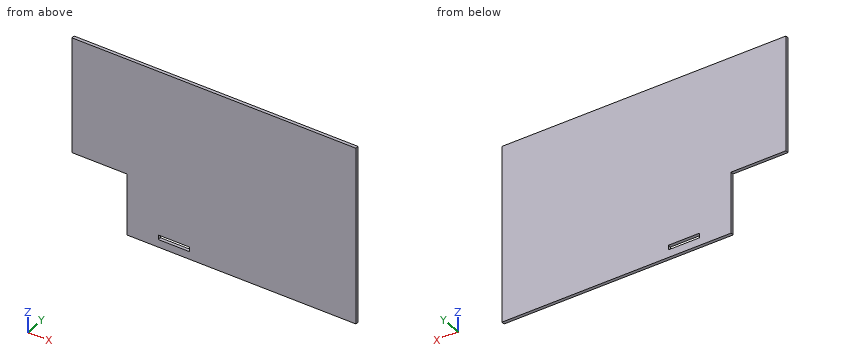
```python
from build123d import *

# Parameters (mm, degrees)
SKETCH1_W           = 25.4
SKETCH1_H           = 3.81
BOSS_EXTRUDE1_DEPTH = 2.54


with BuildPart() as part:
    # Sketch1 → Boss-Extrude1 (new body)
    with BuildSketch(Plane(origin=(0, 0, 0), x_dir=(1, 0, 0), z_dir=(0, 1, 0))):
        Polygon((0, -50.8), (44.45, -50.8), (44.45, 0), (229.87, 0), (229.87, -146.4056), (0, -146.4056), align=None)
        with Locations((82.55, -8.255)):
            Rectangle(SKETCH1_W, SKETCH1_H, mode=Mode.SUBTRACT)
    extrude(amount=BOSS_EXTRUDE1_DEPTH)


solid = part.part
```
Here's how the part is built. I have some questions about the finished solid (model axes, mm). Round coordinates to 2 decimals unless told otherwise and drop trailing zeros. Loops run counter-clockwise (first coordinate to the right, second up) from the corner with the lowest first, then second, coordinate; pieces in that order, holes last.
1. Suppose I cut it at C-C, the plane z = 32.5. Please give me the cut outline in (x, y).
Answers:
outline: (44.45, 0) - (229.87, 0) - (229.87, 2.54) - (44.45, 2.54) - close
2. Suppose I cut it at B-B, the plane x = 89. Please give me the cut outline in (y, z), and give its area (3 significant figures).
Answers:
outline: (0, 0) - (2.54, 0) - (2.54, 6.35) - (0, 6.35) - close; (0, 10.16) - (2.54, 10.16) - (2.54, 146.41) - (0, 146.41) - close
area: 362 mm2
3. Will these pins go through, and if not, where does the flat tip stop? pin 1 (0.8 mm diameter, centred on x = 81, y = 1.5, fed in from -Z); pin 2 (0.8 mm diameter, centred on x = 22.5, y = 2, fed in from -Z); pin 3 (1.3 mm diameter, centred on y = 1.5, z = 33, fed in from -X).
Answers:
pin 1: stops at z = 0
pin 2: stops at z = 50.8
pin 3: stops at x = 44.45
4. If I drill on probe 1 along Z at (x, y) = (73, 1.7); probe 2 along X at (y, z) = (2.2, 15); probe 3 along Z at (x, y) = (17, 0.85), over which ranges is the centre line in solid material (lowest first)?
Answers:
probe 1: z = 0 to 6.35, 10.16 to 146.41
probe 2: x = 44.45 to 229.87
probe 3: z = 50.8 to 146.41
5. Suppose I cut it at A-A, the plane y = 1.55. Please give me the cut outline in (x, z).
Answers:
outline: (0, 50.8) - (44.45, 50.8) - (44.45, 0) - (229.87, 0) - (229.87, 146.41) - (0, 146.41) - close; hole (69.85, 6.35) - (95.25, 6.35) - (95.25, 10.16) - (69.85, 10.16) - close
